Could you check a few things on this model? Use its own coordinates, in mm. Face numbers are marked on the shaded views. Round coordinates to 2 decimals unless told otherwise and drop trailing zeros. Loops run counter-clockwise (first coordinate to the right, second up) from the corner with the lowest first, then second, coordinate; pieces in that order, holes last. Notation, with made-up numbers: (16.25, 4) -> (60.25, 4) arc R18 cw to (60.25, 9) -> close; hole circle Ø8 at (78, 50). An arc over 180 degrees is marked (long way). One line per item, written item: value.
```python
from build123d import *

# Parameters (mm, degrees)
SKETCH1_W               = 31
SKETCH1_H               = 27
BOSS_EXTRUDE1_DEPTH     = 1
SKETCH2_R               = 1.5
BOSS_EXTRUDE2_DEPTH     = 10
MIRROR2_COPY_1_SKETCH_R = 1.5
MIRROR2_COPY_1_DEPTH    = 10


with BuildPart() as part:
    # Sketch1 → Boss-Extrude1 (new body)
    with BuildSketch(Plane.XY):
        Rectangle(SKETCH1_W, SKETCH1_H)
    extrude(amount=BOSS_EXTRUDE1_DEPTH)

    # Sketch2 → Boss-Extrude2 (add)
    with BuildSketch(Plane(origin=(0, 0, 0), x_dir=(-1, 0, 0), z_dir=(0, 0, -1))):
        with Locations((-11.4, -9.4)):
            Circle(SKETCH2_R)
    boss_extrude2 = extrude(amount=BOSS_EXTRUDE2_DEPTH)

    # Mirror1: Boss-Extrude2 across plane
    add(boss_extrude2.mirror(Plane.ZX))

    # Mirror2: Boss-Extrude2 across plane
    add(boss_extrude2.mirror(Plane(origin=(0, 0, 0), x_dir=(0, 0, 1), z_dir=(1, 0, 0))))

    # Mirror2 copy 1 sketch → Mirror2 copy 1 (add)
    with BuildSketch(Plane(origin=(0, 0, 0), x_dir=(1, 0, 0), z_dir=(0, 0, -1))):
        with Locations((-11.4, -9.4)):
            Circle(MIRROR2_COPY_1_SKETCH_R)
    extrude(amount=MIRROR2_COPY_1_DEPTH)


solid = part.part
```
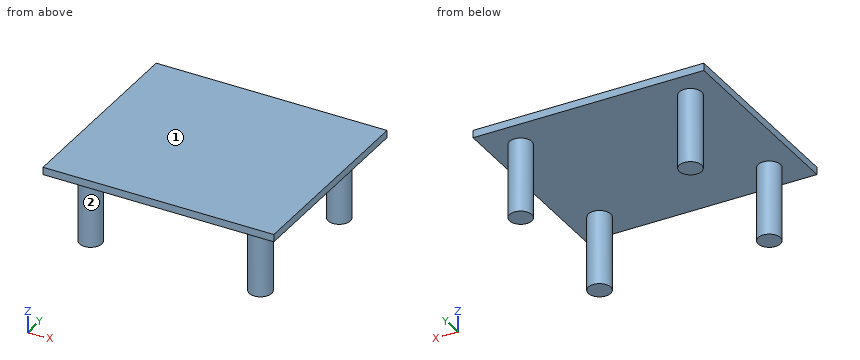
Item 1: If we section it at A-A on x = -11.4: List the corners of the cut face in (y, z) for me.
Output:
outline: (-13.5, 0) -> (-10.9, 0) -> (-10.9, -10) -> (-7.9, -10) -> (-7.9, 0) -> (7.9, 0) -> (7.9, -10) -> (10.9, -10) -> (10.9, 0) -> (13.5, 0) -> (13.5, 1) -> (-13.5, 1) -> close
Item 2: If we mould it in two halves opening along X, with no side actions, what happens to the marked faces 1 and 2? For each: released by +X, released by -X, zero draft, split by the parting line, or undercut.
Output:
face 1: zero draft
face 2: undercut
Item 3: If we section it at C-C on z = -4.75: List the corners of the cut face in (x, y) for me.
Output:
outline: circle Ø3 at (-11.4, -9.4); circle Ø3 at (-11.4, 9.4); circle Ø3 at (11.4, -9.4); circle Ø3 at (11.4, 9.4)
Item 4: If we section it at B-B on y = 9.4: List the corners of the cut face in (x, z) for me.
Output:
outline: (-15.5, 0) -> (-12.9, 0) -> (-12.9, -10) -> (-9.9, -10) -> (-9.9, 0) -> (9.9, 0) -> (9.9, -10) -> (12.9, -10) -> (12.9, 0) -> (15.5, 0) -> (15.5, 1) -> (-15.5, 1) -> close
Item 5: I need wall thicknesses on line 1 (X direction, y = 9.25, z = -7.75); line 2 (Z direction, x = 5, y = 10.75); line 3 (X direction, y = -10, z = -2.25). Which ranges of each line are inside material? Lowest first, please. Write a range as from..to.
Output:
line 1: x = -12.89..-9.91, 9.91..12.89
line 2: z = 0..1
line 3: x = -12.77..-10.03, 10.03..12.77
Item 6: Will these pins go through, and if not, where does the flat tip stop? pin 1 Ø8 at (x, y) = (3, -1) entering from -Z; pin 2 Ø3 at (x, z) = (9, -5) entering from -Y; pin 3 Ø2 at (y, z) = (-9, -2) entering from -X.
Output:
pin 1: stops at z = 0
pin 2: stops at y = -10.6
pin 3: stops at x = -12.9
